```python
from build123d import *

# Parameters (mm, degrees)
SKETCH_1_W          = 10
SKETCH_1_H          = 15
SKETCH_1_W_2        = 7
SKETCH_1_H_2        = 12
EXTRUDE_1_DEPTH     = 600
SKETCH_2_R          = 1.6
CUT_EXTRUDE_1_DEPTH = 601.208297177
SKETCH_3_R          = 1.6
CUT_EXTRUDE_2_DEPTH = 601.130194208


with BuildPart() as part:
    # ｽｹｯﾁ1 → 押し出し-薄板1 (new body)
    with BuildSketch(Plane.XY):
        Rectangle(SKETCH_1_W, SKETCH_1_H)
        Rectangle(SKETCH_1_W_2, SKETCH_1_H_2, mode=Mode.SUBTRACT)
    extrude(amount=EXTRUDE_1_DEPTH)

    # ｽｹｯﾁ2 → ｶｯﾄ - 押し出し1 (cut, through all)
    with BuildSketch(Plane(origin=(0, 7.5, 0), x_dir=(1, 0, 0), z_dir=(0, 1, 0))):
        with Locations(Location((0, -595, 0), (0, 0, 270))):
            Circle(SKETCH_2_R)
        with Locations(Location((0, -5, 0), (0, 0, 270))):
            Circle(SKETCH_2_R)
        with Locations(Location((0, -500, 0), (0, 0, 270))):
            Circle(SKETCH_2_R)
        with Locations(Location((0, -100, 0), (0, 0, 270))):
            Circle(SKETCH_2_R)
    extrude(amount=-CUT_EXTRUDE_1_DEPTH, mode=Mode.SUBTRACT)

    # ｽｹｯﾁ3 → ｶｯﾄ - 押し出し2 (cut, through all)
    with BuildSketch(Plane(origin=(5, 0, 0), x_dir=(0, 0, -1), z_dir=(1, 0, 0))):
        with Locations((-585, 0)):
            Circle(SKETCH_3_R)
        with Locations((-15, 0)):
            Circle(SKETCH_3_R)
        with Locations((-490, 0)):
            Circle(SKETCH_3_R)
        with Locations((-110, 0)):
            Circle(SKETCH_3_R)
    extrude(amount=-CUT_EXTRUDE_2_DEPTH, mode=Mode.SUBTRACT)


solid = part.part
```
Build history of the part. All positions in model axes, mm. Give positions to 0.01 mm unless a question says otherwise; leave off trailing zeros. Order: outer loops, then holes, each group sorted by start corner. A loop starts at its lowest first (then second) coordinate and runs counter-clockwise, first axis right, second up. Notation, with made-up numbers: M 72.5,-36.75 L 121.5,-36.75 A27 ccw 121.5,-15.75 Z; hole C 82,-37 d4. An arc over 180 degrees is marked long. Return JSON: item names as keys, results as strings.
Q1. Wall check: probe 1 along X at (y, z) = (0.75, 540); probe 2 along Y at (x, z) = (-3, 438.5); probe 3 along Y at (x, z) = (4.1, 585). Give the ranges that are in metal, low to high. Write a range as from..to.
Answer list:
{"probe 1": "x = -5..-3.5, 3.5..5", "probe 2": "y = -7.5..-6, 6..7.5", "probe 3": "y = -7.5..-1.6, 1.6..7.5"}
Q2. Two-plate mould, pull along Y, no slides. Class faces 1 (the face through (3.5, 0, 296)), 2 (the face through (-3.5, 0, 296)), 3 (the face through (-5, 0, 296)), 4 (the face through (0, 7.5, 296)): pulls with the +Y half, pulls with the -Y half, needs draft (parallel to the pull), parting line crosses it, or undercut.
Answer list:
{"face 1": "undercut", "face 2": "undercut", "face 3": "needs draft", "face 4": "pulls with the +Y half"}
Q3. Band-saw the part on A-A (z = 422.5). Give the cut face in (x, y).
Answer list:
{"outline": "M -5,-7.5 L 5,-7.5 L 5,7.5 L -5,7.5 Z; hole M -3.5,-6 L 3.5,-6 L 3.5,6 L -3.5,6 Z"}
